Could you check a few things on this drawing? It's one solid part, dimensions in mm from its lowest x, y, z. Round coordinates to 2 decimals unless told otherwise and drop trailing zeros. Loops run counter-clockwise (first coordinate to the right, second up) from the corner with the lowest first, then second, coordinate; pieces in that order, holes last. Notation, with made-up numbers: M 65.25,24 L 121.25,24 A19 ccw 121.25,45 Z; hole C -1,-4 d7. An arc over 180 degrees is marked long. Answer as a JSON object with one key per item and string values.
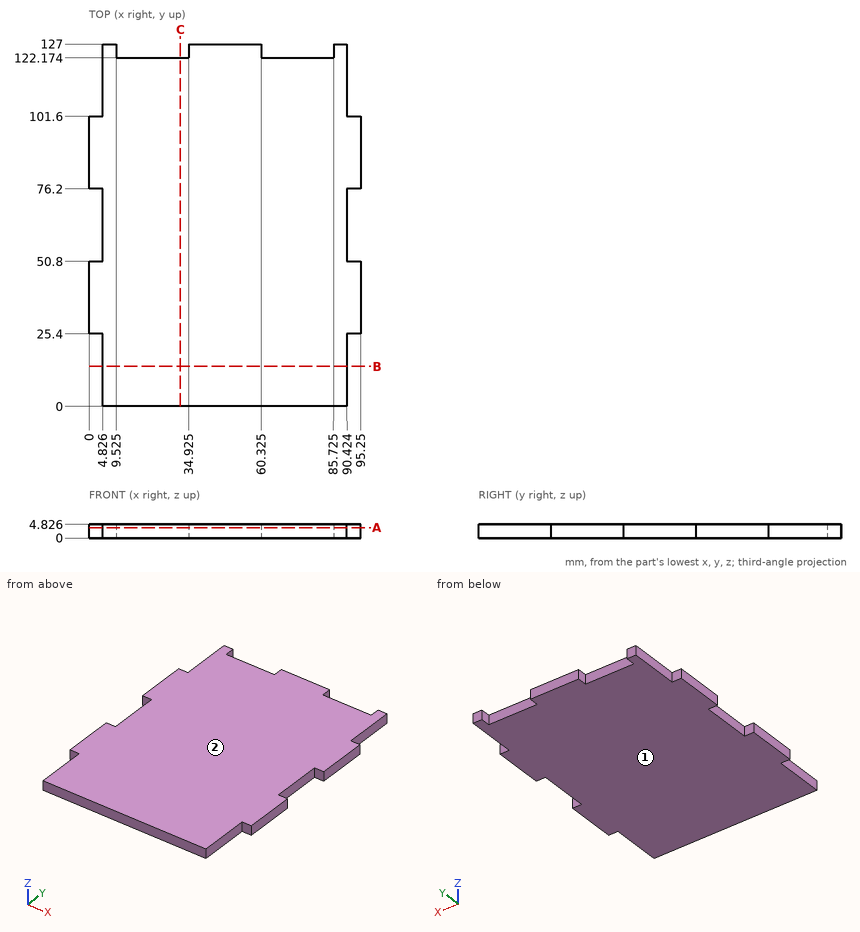
Item 1: I want a section at A-A, the plane z = 3.65. Please give me the cut outline in (x, y) (3 decimals).
Resolved:
{"outline": "M 0,25.4 L 4.826,25.4 L 4.826,0 L 90.424,0 L 90.424,25.4 L 95.25,25.4 L 95.25,50.8 L 90.424,50.8 L 90.424,76.2 L 95.25,76.2 L 95.25,101.6 L 90.424,101.6 L 90.424,127 L 85.725,127 L 85.725,122.174 L 60.325,122.174 L 60.325,127 L 34.925,127 L 34.925,122.174 L 9.525,122.174 L 9.525,127 L 4.826,127 L 4.826,101.6 L 0,101.6 L 0,76.2 L 4.826,76.2 L 4.826,50.8 L 0,50.8 Z"}
Item 2: I'm going to push flat-ended pins straight in: pin 1 Ø1.4 at (x, z) = (92.5, 2.5) entering from -Y; pin 2 Ø2.5 at (y, z) = (125, 2.5) entering from +X; pin 3 Ø1.4 at (y, z) = (65.5, 3.5) entering from -X. Where does each tip first touch, or does it pass through?
Resolved:
{"pin 1": "y = 25.4", "pin 2": "x = 90.42", "pin 3": "x = 4.83"}
Item 3: I want a section at C-C, the plane x = 32. Please give me the cut outline in (y, z).
Resolved:
{"outline": "M 0,0 L 122.17,0 L 122.17,4.83 L 0,4.83 Z"}
Item 4: I want a section at B-B, the plane y = 14. Please give me the cut outline in (x, z), then the cut area to 3 significant figures.
Resolved:
{"outline": "M 4.83,0 L 90.42,0 L 90.42,4.83 L 4.83,4.83 Z", "area": "413 mm²"}
Item 5: If we mould it in two halves opening along Z, with no side actions, what happens to the marked faces 1 and 2? For each: pulls with the +Z half, pulls with the -Z half, needs draft (parallel to the pull), parting line crosses it, or undercut.
Resolved:
{"face 1": "pulls with the -Z half", "face 2": "pulls with the +Z half"}
Item 6: Please list where these lines run through material, in increasing order: probe 1 along Y at (x, z) = (75, 2.9); probe 2 along X at (y, z) = (121.5, 2.65). Write a range as from..to.
Resolved:
{"probe 1": "0..122.17", "probe 2": "4.83..90.42"}
